Job drawing, mm, ordinate dimensions from the low corner. One solid piece. Coordinates: 2 decimals unless noted, no trailing zeros. Order: outer loops, then holes, each group sorted by start corner. A loop starts at its lowest first (then second) coordinate and runs counter-clockwise, first axis right, second up. Notation, with made-up numbers: (-22, 33) - (11, 33) arc R24 cw to (11, 67) - close; hole circle Ø4 at (30, 47). An arc over 180 degrees is marked (long way). Use one line per item in the form item = value.
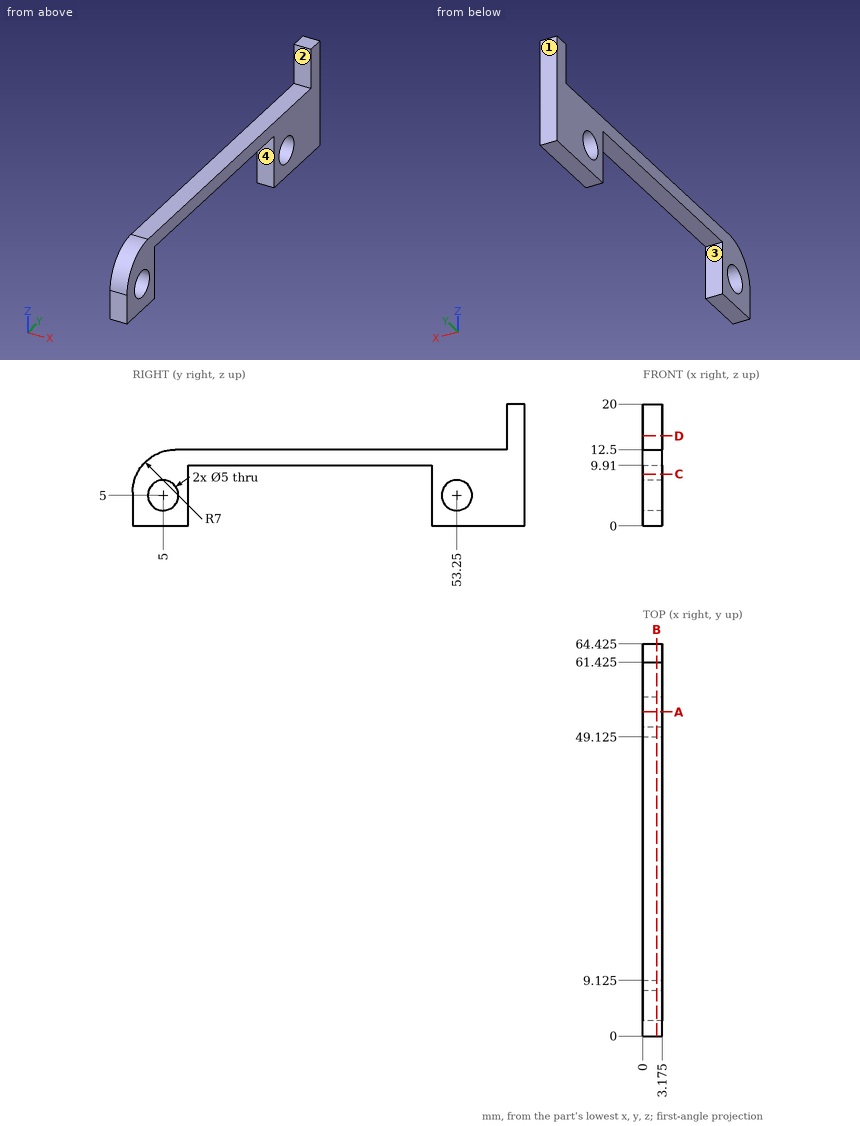
Item 1: Cut at C-C, the plane z = 8.5. Write the cut outline in (x, y) (3 decimals), plus the area to 3 significant figures.
Derived:
outline = (0, 0.675) - (3.175, 0.675) - (3.175, 9.125) - (0, 9.125) - close; (0, 49.125) - (3.175, 49.125) - (3.175, 64.425) - (0, 64.425) - close
area = 75.4 mm²
Item 2: Cut at D-D, the plane z = 14.75. Write the cut outline in (x, y) (3 decimals).
Derived:
outline = (0, 61.425) - (3.175, 61.425) - (3.175, 64.425) - (0, 64.425) - close
Item 3: Drill centre lines: line 1 (Y direction, x = 2.8, z = 5.25) (3 decimals); line 2 (Z direction, x = 1.8, y = 53); line 3 (Y direction, x = 1.25, z = 4.25) (3 decimals). Where is each one in solid material? Low to high. Write a range as [from, to].
Derived:
line_1 = [0, 2.513], [7.487, 9.125], [49.125, 50.763], [55.737, 64.425]
line_2 = [0, 2.51], [7.49, 12.5]
line_3 = [0, 2.615], [7.385, 9.125], [49.125, 50.865], [55.635, 64.425]
Item 4: Cut at B-B, the plane x = 2.25. Write the cut outline in (y, z) (3 decimals), plus the area to 3 significant figures.
Derived:
outline = (0, 0) - (9.125, 0) - (9.125, 9.91) - (49.125, 9.91) - (49.125, 0) - (64.425, 0) - (64.425, 20) - (61.425, 20) - (61.425, 12.5) - (7, 12.5) arc R7 ccw to (0, 5.5) - close; hole circle Ø5 at (5, 5); hole circle Ø5 at (53.25, 5)
area = 382 mm²
Item 5: Two-plate mould, pull along Y, no slides. Class the marked faces 1, 2, 3 and 4: +Y half, -Y half, draft (parallel to the pull), parting line (faces both ways), or undercut.
Derived:
face_1 = +Y half
face_2 = -Y half
face_3 = undercut
face_4 = undercut
Item 6: Drop a flat-ended pin along its axis: pin 1 (4 mm diameter, centred on y = 53.25, z = 5, fed in from -X). Give the stop position or say it passes through.
Derived:
pin_1 = through
Item 7: Cut at A-A, the plane y = 53.25. Write the cut outline in (x, z) (3 decimals), plus the area to 3 significant figures.
Derived:
outline = (0, 0) - (3.175, 0) - (3.175, 2.5) - (0, 2.5) - close; (0, 7.5) - (3.175, 7.5) - (3.175, 12.5) - (0, 12.5) - close
area = 23.8 mm²
